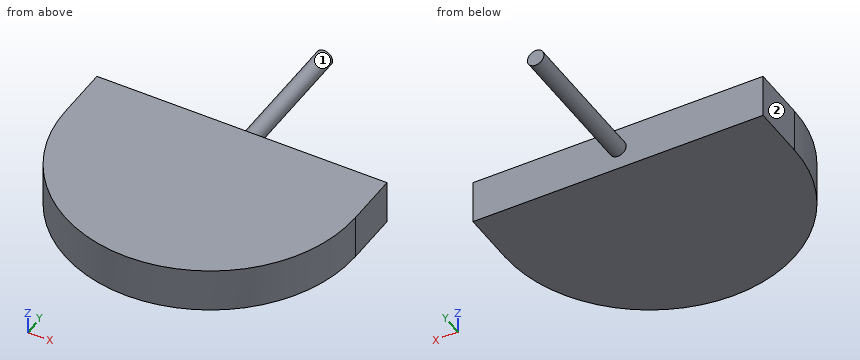
```python
from build123d import *

# Parameters (mm, degrees)
BOSS_EXTRUDE1_DEPTH = 3.99
SKETCH2_R           = 0.75
BOSS_EXTRUDE2_DEPTH = 13.019979


with BuildPart() as part:
    # Sketch1 → Boss-Extrude1 (new body)
    with BuildSketch(Plane.XY):
        with BuildLine():
            Line((-13.2, -2.5), (-13.2, 2.5))
            Line((-13.2, 2.5), (13.2, 2.5))
            Line((13.2, 2.5), (13.2, -2.5))
            ThreePointArc((13.2, -2.5), (0, -15.7), (-13.2, -2.5))
        make_face()
    extrude(amount=BOSS_EXTRUDE1_DEPTH)

    # Sketch2 → Boss-Extrude2 (add)
    with BuildSketch(Plane(origin=(0, 2.5, 0), x_dir=(1, 0, 0), z_dir=(0, 1, 0))):
        with Locations((0, -1.995)):
            Circle(SKETCH2_R)
    extrude(amount=BOSS_EXTRUDE2_DEPTH)


solid = part.part
```
Can you work these out from the model? Positions are in its coordinate system, mm. Face numbers are marked on the shaded views. A direction names the side the tool comes from. Coordinates: 2 decimals unless noted, no trailing zeros. Order: outer loops, then holes, each group sorted by start corner. A loop starts at its lowest first (then second) coordinate and runs counter-clockwise, first axis right, second up. Notation, with made-up numbers: (10, 20.5) - (59, 20.5) arc R21 cw to (59, 55.5) - close; hole circle Ø2 at (-6.5, 39). An arc over 180 degrees is marked (long way). Answer in a Markdown table with one row per item.
1. For the marked faces 1 and 2, which set-ups out of +Z, -Z, +X, -X, +Y, -Y let a thin tool reach every point of the face, with its end or its side?
Reply:
| item | result |
|---|---|
| face 1 | +Y |
| face 2 | +Z, -Z, -X, +Y, -Y |
2. Suppose I cut it at B-B (z = 1.65). Please give me the cut outline in (x, y), and give its area (3 significant figures).
Reply:
| item | result |
|---|---|
| outline | (-13.2, -2.5) arc R13.2 ccw to (13.2, -2.5) - (13.2, 2.5) - (0.67, 2.5) - (0.67, 15.52) - (-0.67, 15.52) - (-0.67, 2.5) - (-13.2, 2.5) - close |
| area | 423 mm^2 |
3. Suppose I cut it at A-A (x = 0). Please give me the cut outline in (y, z) (3 decimals).
Reply:
| item | result |
|---|---|
| outline | (-15.7, 0) - (2.5, 0) - (2.5, 1.245) - (15.52, 1.245) - (15.52, 2.745) - (2.5, 2.745) - (2.5, 3.99) - (-15.7, 3.99) - close |
4. For pin 1 (2 mm diameter, centred on y = 6.5, z = 1.5, fed in from +X); pin 2 (1.5 mm diameter, centred on x = 3, z = 2.5, fed in from -Y); pin 3 (2 mm diameter, centred on x = -8, z = 2.5, fed in from +Y), each with a flat end and sliding along its axis, tell me the tip position at first contact or that it passes through.
Reply:
| item | result |
|---|---|
| pin 1 | stops at x = 0.75 |
| pin 2 | stops at y = -15.51 |
| pin 3 | stops at y = 2.5 |
5. Suppose I cut it at D-D (x = 3). Please give me the cut outline in (y, z), and give its area (3 significant figures).
Reply:
| item | result |
|---|---|
| outline | (-15.35, 0) - (2.5, 0) - (2.5, 3.99) - (-15.35, 3.99) - close |
| area | 71.2 mm^2 |
6. If I drill on line 1 along X through (y, z) = (9.5, 1.9); line 2 along Y through (x, z) = (-1.25, 3.3); line 3 along Y through (x, z) = (11, 3.6), over which ranges is the centre line in solid material (lowest first)?
Reply:
| item | result |
|---|---|
| line 1 | x = -0.74 to 0.74 |
| line 2 | y = -15.64 to 2.5 |
| line 3 | y = -9.8 to 2.5 |
7. Suppose I cut it at C-C (y = 8). Please give me the cut outline in (x, z) (3 decimals).
Reply:
| item | result |
|---|---|
| outline | circle Ø1.5 at (0, 1.995) |
